Part model, mm, in its own coordinate system. A direction names the side the tool comes from. Give positions to 0.01 mm unless a question says otherwise; leave off trailing zeros. Write each loop counter-clockwise with the first axis right and the second up, starting at its lowest first coordinate (ties: lowest second). Pieces come first, ordered by that corner, then holes.
from build123d import *

# Parameters (mm, degrees)
F1_DEPTH  = 800
F3_DEPTH  = 25
F4_W      = 1255.690882
F4_H      = 80
F5_DEPTH  = 25
F6_R      = 60
F6_R_2    = 100
F7_DEPTH  = 25
F9_DEPTH  = 10
F11_DEPTH = 487


with BuildPart() as f1:
    # F0 (on Top) → F1 (new body)
    with BuildSketch(Plane.XY):
        Polygon((-500, 500), (-500, -500), (500, -500), (500, 100), (100, 500), align=None)
    extrude(amount=F1_DEPTH)

    # F2 (on face) → F3 (join)
    with BuildSketch(Plane.XY.offset(800)):
        Polygon((-500, 500), (-500, -500), (500, -500), (500, 125), (125, 500), align=None)
    extrude(amount=F3_DEPTH)

    # F4 (on face) → F5 (cut)
    with BuildSketch(Plane(origin=(300, 300, 0), x_dir=(-0.707107, 0.707107, 0), z_dir=(0.707107, 0.707107, 0))):
        with Locations((133.201046, 40)):
            Rectangle(F4_W, F4_H)
    extrude(amount=-F5_DEPTH, mode=Mode.SUBTRACT)

    # F6 (on face) → F7 (join)
    with BuildSketch(Plane.XY.offset(825)):
        with Locations((241.789322, 241.789322)):
            Circle(F6_R)
        with Locations((94.470174, 94.470174)):
            Circle(F6_R)
        with Locations((347.855339, -5.698052)):
            Circle(F6_R_2)
        with Locations((-5.698052, 347.855339)):
            Circle(F6_R_2)
    extrude(amount=F7_DEPTH)

    # F8 (on face) → F9 (cut)
    with BuildSketch(Plane(origin=(300, 300, 0), x_dir=(-0.707107, 0.707107, 0), z_dir=(0.707107, 0.707107, 0))):
        with BuildLine():
            ThreePointArc((-182.842712, 310), (-174.055916, 288.786797), (-152.842712, 280))
            Line((-152.842712, 280), (152.842712, 280))
            ThreePointArc((152.842712, 280), (174.055916, 288.786797), (182.842712, 310))
            Line((182.842712, 310), (182.842712, 600))
            ThreePointArc((182.842712, 600), (174.055916, 621.213203), (152.842712, 630))
            Line((152.842712, 630), (-152.842712, 630))
            ThreePointArc((-152.842712, 630), (-174.055916, 621.213203), (-182.842712, 600))
            Line((-182.842712, 600), (-182.842712, 310))
        make_face()
    extrude(amount=-F9_DEPTH, mode=Mode.SUBTRACT)

    # F10 (on face) → F11 (join)
    with BuildSketch(Plane.XY.offset(825)):
        Polygon((-500, 200), (-500, -500), (200, -500), align=None)
    extrude(amount=F11_DEPTH)


solid = f1.part
1) Saw through at B-B (y = -322). Write the cut outline in (x, z).
Check result:
outline: (-500, 0) - (500, 0) - (500, 825) - (22, 825) - (22, 1312) - (-500, 1312) - close
2) Saw through at A-A (z = 460.5). Write the cut outline in (x, y), and give its area (3 significant figures).
Check result:
outline: (-500, -500) - (500, -500) - (500, 100) - (429.29, 170.71) - (422.22, 163.64) - (163.64, 422.22) - (170.71, 429.29) - (100, 500) - (-500, 500) - close
area: 916,000 mm2
3) Drill centre lines: L1, parallel to Z at x = -196.5, y = 128; L2, parallel to Z at x = -43.5, y = 312; L3, parallel to X at y = 251.5, z = 135. Where is each one in solid material? Low to high.
Check result:
L1: z = 0 to 825
L2: z = 0 to 850
L3: x = -500 to 348.5
4) Mould opens along Y. For faces 1 (the flat face through (285.37, 279.275, 40.56)), 2 (the cylindrical face through (-18.716, 447.004, 837.325)), 3 (the flat face through (-7, -500, 647)), 4 (the flat face through (294, 288, 80)) say: +Y half, -Y half, draft (parallel to the pull), parting line (faces both ways), or undercut.
Check result:
face 1: +Y half
face 2: undercut
face 3: -Y half
face 4: draft
5) 3-axis set-ups, long thin cutter, end or side, ignore diameter. For faces 5 (the flat face through (299, 316, 800)), 6 (the flat face through (346, -4, 850)), 7 (the flat face through (94, 95, 850)), 8 (the flat face through (298, 295, 280)), 9 (the cylindrical face through (122.16, 41.24, 837.32)): which of +Z, -Z, +X, -X, +Y, -Y reach the whole face in a straight line?
Check result:
face 5: -Z, +X, +Y
face 6: +Z, +X, +Y, -Y
face 7: +Z, +X, +Y
face 8: +X, +Y
face 9: +Z
6) Flat gauge pins, fed straight in: P1, Ø12, axis at x = 280, y = 325, coming from the +Z side; P2, Ø10, axis at y = 259, z = 772, coming from the +X side; P3, Ø4, axis at x = 241.5, z = 790, coming from the +Y side. Where does each tip first touch, or does it go through?
Check result:
P1: stops at z = 825
P2: stops at x = 346
P3: stops at y = 360.5
7) Saw through at D-D (z = 129). Write the cut outline in (x, y), and give its area (3 significant figures).
Check result:
outline: (-500, -500) - (500, -500) - (500, 100) - (100, 500) - (-500, 500) - close
area: 920,000 mm2
8) Saw through at C-C (x = -269). Write the cut outline in (y, z).
Check result:
outline: (-500, 0) - (500, 0) - (500, 825) - (-31, 825) - (-31, 1312) - (-500, 1312) - close
